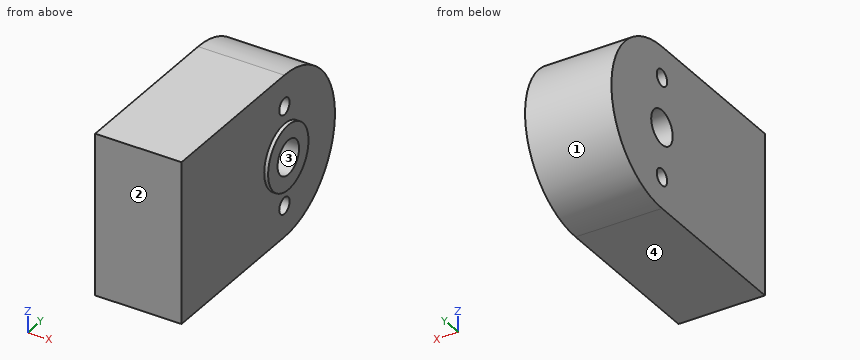
```python
from build123d import *

# Parameters (mm, degrees)
BOSS_EXTRUDE1_DEPTH = 16.59
SKETCH2_R           = 6.2
BOSS_EXTRUDE2_DEPTH = 0.75
SKETCH3_R           = 3.3
SKETCH3_R_2         = 1.5875
CUT_EXTRUDE1_DEPTH  = 40.258240536


with BuildPart() as part:
    # Sketch1 → Boss-Extrude1 (new body)
    with BuildSketch(Plane(origin=(0, 0, 0), x_dir=(0, 0, -1), z_dir=(1, 0, 0))):
        with BuildLine():
            Line((-15.525, -31.615), (15.525, -31.615))
            Line((15.525, -31.615), (15.525, 0))
            ThreePointArc((15.525, 0), (0, 15.525), (-15.525, 0))
            Line((-15.525, 0), (-15.525, -31.615))
        make_face()
    extrude(amount=BOSS_EXTRUDE1_DEPTH)

    # Sketch2 → Boss-Extrude2 (add)
    with BuildSketch(Plane(origin=(16.59, 0, 0), x_dir=(0, 0, -1), z_dir=(1, 0, 0))):
        with Locations(Location((0, 0, 0), (0, 0, 180))):
            Circle(SKETCH2_R)
    extrude(amount=BOSS_EXTRUDE2_DEPTH)

    # Sketch3 → Cut-Extrude1 (cut, through all)
    with BuildSketch(Plane(origin=(17.34, 0, 0), x_dir=(0, 0, -1), z_dir=(1, 0, 0))):
        Circle(SKETCH3_R)
        with Locations((-9.525, 0)):
            Circle(SKETCH3_R_2)
        with Locations((9.525, 0)):
            Circle(SKETCH3_R_2)
    extrude(amount=-CUT_EXTRUDE1_DEPTH, mode=Mode.SUBTRACT)


solid = part.part
```
Here's how the part is built. I have some questions about the finished solid (model axes, mm). Face numbers are marked on the shaded views. Coordinates: 2 decimals unless noted, no trailing zeros. Write each loop counter-clockwise with the first axis right and the second up, starting at its lowest first coordinate (ties: lowest second). Pieces come first, ordered by that corner, then holes. Notation, with made-up numbers: (-20, -7.5) -> (30, -7.5) arc R19 ccw to (30, -0.5) -> close; hole circle Ø8 at (28.25, 60.5). An arc over 180 degrees is marked (long way). Use a Markdown table: item, result. Add a question column.
(1) I'm going to push flat-ended pins straight in: P1, Ø5, axis at y = -2, z = 6, coming from the +X side; P2, Ø6, axis at y = -26, z = -8, coming from the +X side; P3, Ø4, axis at y = 0, z = 0, coming from the +X side; P4, Ø3, axis at x = 13.5, z = 5.5, coming from the +Y side. Where does each tip first touch, or does it pass through?
(2) If we section it at B-B, the plane x = 8.5: State how many separate pieces and enclosed holes the cut face has, and give its area (3 significant figures).
(3) If we section it at A-A, the plane z = 0: Write out the boundary of the cut face in (x, y) (3 decimals).
(4) Please list where these lines run through material, in increasing order: line 1 (Y direction, x = 4.75, z = 0) (3 decimals); line 2 (X direction, y = -12, z = 8.5); line 3 (Y direction, x = 13.25, z = -1) (3 decimals).
(5) If we section it at C-C, the plane z = 8.5: Write out the boundary of the cut face in (x, y) (3 decimals), and give its area (3 significant figures).
(6) We'd pull the mould along Y, two halves only. Please class the marked faces 1, 2, 3 and 4: +Y half, -Y half, draft (parallel to the pull), parting line (faces both ways), or undercut.
(7) If we section it at D-D, the plane y = -22.5: Write out the boundary of the cut face in (x, z) (3 decimals), and give its area (3 significant figures).
Outcome:
| question | item | result |
|---|---|---|
| 1 | P1 | stops at x = 17.34 |
| 1 | P2 | stops at x = 16.59 |
| 1 | P3 | passes through |
| 1 | P4 | stops at y = 15 |
| 2 | separate pieces | 1 |
| 2 | enclosed holes | 3 |
| 2 | area | 1,310 mm^2 |
| 3 | outline | (0, -31.615) -> (16.59, -31.615) -> (16.59, -6.2) -> (17.34, -6.2) -> (17.34, -3.3) -> (0, -3.3) -> close; (0, 3.3) -> (17.34, 3.3) -> (17.34, 6.2) -> (16.59, 6.2) -> (16.59, 15.525) -> (0, 15.525) -> close |
| 4 | line 1 | y = -31.615 to -3.3, 3.3 to 15.525 |
| 4 | line 2 | x = 0 to 16.59 |
| 4 | line 3 | y = -31.615 to -3.145, 3.145 to 15.493 |
| 5 | outline | (0, -31.615) -> (16.59, -31.615) -> (16.59, -1.212) -> (0, -1.212) -> close; (0, 1.212) -> (16.59, 1.212) -> (16.59, 12.991) -> (0, 12.991) -> close |
| 5 | area | 700 mm^2 |
| 6 | face 1 | +Y half |
| 6 | face 2 | -Y half |
| 6 | face 3 | undercut |
| 6 | face 4 | draft |
| 7 | outline | (0, -15.525) -> (16.59, -15.525) -> (16.59, 15.525) -> (0, 15.525) -> close |
| 7 | area | 515 mm^2 |
